Job drawing, mm, ordinate dimensions from the low corner. One solid piece. Give positions to 0.01 mm unless a question says otherwise; leave off trailing zeros. Loops run counter-clockwise (first coordinate to the right, second up) from the corner with the lowest first, then second, coordinate; pieces in that order, holes last.
Item 1: Saw through at A-A on z = 2. Give the cut face in (x, y).
Item 2: Drop a flat-ended pin along its axis: P1, Ø1.5, axis at x = 2.5, z = 2.5, coming from the +Y side. Give the stop position or say it passes through.
Item 3: Mould opens along X. For the marked faces 1, 2 and 3 say: released by +X, released by -X, zero draft, split by the parting line, or undercut.
Item 4: Probe probe 1 along Y at (x, z) = (4, 1.65); probe 2 along Y at (x, z) = (3.5, 0.8); probe 3 along X at (y, z) = (2.5, 1.9). List the from-to ranges inside material, lowest first.
Item 5: Saw through at B-B on y = 1. Give the cut face in (x, z), plus the area to 3 significant figures.
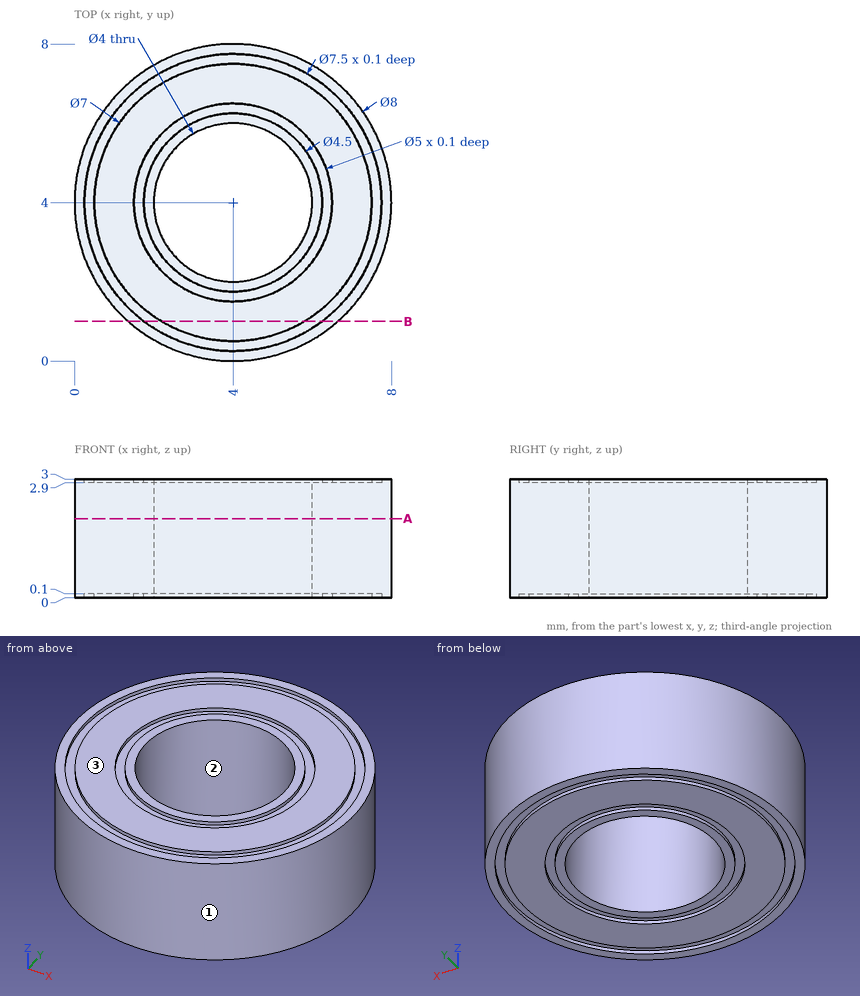
Results below:
1. outline: circle Ø8 at (4, 4); hole circle Ø4 at (4, 4)
2. P1: stops at y = 7.93
3. face 1: split by the parting line
3. face 2: undercut
3. face 3: zero draft
4. probe 1: y = 0 to 2, 6 to 8
4. probe 2: y = 0.03 to 2.06, 5.94 to 7.97
4. probe 3: x = 0.29 to 2.68, 5.32 to 7.71
5. outline: (1.35, 0) - (1.75, 0) - (1.75, 0.1) - (2.2, 0.1) - (2.2, 0) - (5.8, 0) - (5.8, 0.1) - (6.25, 0.1) - (6.25, 0) - (6.65, 0) - (6.65, 3) - (6.25, 3) - (6.25, 2.9) - (5.8, 2.9) - (5.8, 3) - (2.2, 3) - (2.2, 2.9) - (1.75, 2.9) - (1.75, 3) - (1.35, 3) - close
5. area: 15.7 mm2
